CAD build for the part. Positions are in the model's coordinates, mm. Face numbers are marked on the shaded views. Give positions to 0.01 mm unless a question says otherwise; leave off trailing zeros. Write each loop counter-clockwise with the first axis right and the second up, starting at its lowest first coordinate (ties: lowest second). Pieces come first, ordered by that corner, then holes. Notation, with made-up numbers: (44.5, 71.25) - (89.5, 71.25) arc R24 cw to (89.5, 81.25) - close; hole circle Ø4 at (68, 41). An arc over 180 degrees is marked (long way). Answer as a JSON object with one key per item and string values.
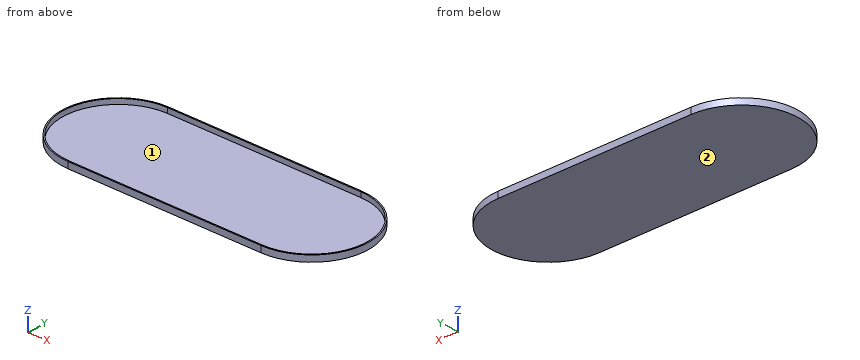
from build123d import *

# Parameters (mm, degrees)
F1_DEPTH = 6.35
F2_T     = -1.27


with BuildPart() as f1:
    # F0 (on Top) → F1 (new body)
    with BuildSketch(Plane.XY):
        with BuildLine():
            Line((0, 57.15), (-196.6468, 57.15))
            ThreePointArc((-196.6468, 57.15), (-253.7968, 0), (-196.6468, -57.15))
            Line((-196.6468, -57.15), (0, -57.15))
            ThreePointArc((0, -57.15), (57.15, 0), (0, 57.15))
        make_face()
    extrude(amount=F1_DEPTH)

    # F2
    f2_openings = [f1.faces().sort_by_distance(p)[0] for p in [
        (-98.3234, 0, 6.35),
    ]]
    offset(amount=F2_T, openings=f2_openings)


solid = f1.part
Item 1: Mould opens along Y. For the marked faces 1 and 2 say: +Y half, -Y half, draft (parallel to the pull), parting line (faces both ways), or undercut.
Entries:
{"face 1": "undercut", "face 2": "draft"}
Item 2: Cut at B-B (z = 2.5). Give the cut face in (x, y), and give its area (3 significant figures).
Entries:
{"outline": "(-196.65, -57.15) - (0, -57.15) arc R57.15 ccw to (0, 57.15) - (-196.65, 57.15) arc R57.15 ccw to start; hole (-196.65, -55.88) - (0, -55.88) arc R55.88 ccw to (0, 55.88) - (-196.65, 55.88) arc R55.88 ccw to start", "area": "950 mm2"}
Item 3: Probe line 1 (Y direction, x = -64, z = 5); line 2 (Y direction, x = 2.5, z = 5.75); line 3 (Z direction, x = -151, y = 38). List the from-to ranges inside material, lowest first. Write a range as from..to.
Entries:
{"line 1": "-57.15..-55.88, 55.88..57.15", "line 2": "-57.1..-55.82, 55.82..57.1", "line 3": "0..1.27"}
Item 4: Cut at C-C (x = -19.5). Give the cut face in (y, z).
Entries:
{"outline": "(-57.15, 0) - (57.15, 0) - (57.15, 6.35) - (55.88, 6.35) - (55.88, 1.27) - (-55.88, 1.27) - (-55.88, 6.35) - (-57.15, 6.35) - close"}
Item 5: Flat gauge pins, fed straight in: P1, Ø1, axis at y = -31, z = 3, coming from the +X side; P2, Ø5, axis at x = -205.5, y = -17.5, coming from the +Z side; P3, Ø1.5, axis at y = 25, z = 1, coming from the -X side. Where does each tip first touch, or does it go through?
Entries:
{"P1": "x = 48.33", "P2": "z = 1.27", "P3": "x = -248.4"}
Item 6: Cut at A-A (y = 0). Give the cut face in (x, z).
Entries:
{"outline": "(-253.8, 0) - (57.15, 0) - (57.15, 6.35) - (55.88, 6.35) - (55.88, 1.27) - (-252.53, 1.27) - (-252.53, 6.35) - (-253.8, 6.35) - close"}
